Part model, mm, in its own coordinate system. A direction names the side the tool comes from. Coordinates: 2 decimals unless noted, no trailing zeros. Write each loop counter-clockwise with the first axis right and the second up, starting at its lowest first coordinate (ties: lowest second). Pieces come first, ordered by that corner, then holes. Notation, with made-up numbers: (89.5, -37.5) -> (113.5, -37.5) arc R17 cw to (113.5, -8.5) -> close; hole circle Ø3 at (70, 34.25). An arc over 180 degrees is marked (long way). One line per question, with ' | ' between items. Start each with the question number.
Item 1: Probe probe 1 along Y at (x, z) = (27, 27); probe 2 along Z at (x, y) = (30, 3.35); probe 3 along Y at (x, z) = (32, 24.5). List the from-to ranges inside material, lowest first. Write a range as [from, to].
Item 2: Two-plate mould, pull along Z, no slides. Class faces 4 (the cylindrical face through (18.894, 23.26, -27.671)), 5 (the flat face through (20, 0, -25)), 6 (the flat face through (20, 0, 25)): pulls with the +Z half, pulls with the -Z half, needs draft (parallel to the pull), parting line crosses it, or undercut.
Item 3: Saw through at C-C (y = 10). List the corners of the cut face in (x, z), and give its area (3 significant figures).
Item 4: Saw through at B-B (x = 30). Count the separate pieces of the cut face and the enclosed holes in it, and give its area (3 significant figures).
Item 5: Saw through at A-A (y = -13). List the corners of the cut face in (x, z), and give its area (3 significant figures).
Item 6: 3-axis set-ups, long thin cutter, end or side, ignore diameter. For faces 1 (the flat face through (20, -6, -11)), 2 (the flat face through (20, 33, 4.5)), 3 (the cylindrical face through (9.675, -36.464, -3.12)): which of +Z, -Z, +X, -X, +Y, -Y reach the whole face in a straight line?
Item 7: Pin check, flat tips, straight feed: pin 1 (3.5 mm diameter, centred on x = 10, y = 35, fed in from +Z); pin 2 (3 mm diameter, centred on x = 17, y = -35, fed in from -Z); pin 3 (4 mm diameter, centred on x = 8, z = 36, fed in from +Y). Stop position of each tip, or through.
from build123d import *

# Parameters (mm, degrees)
SKETCH1_R               = 17.5
SKETCH1_R_2             = 4.75
MAINBODY_DEPTH          = 40
SKETCH2_R               = 17.5
SKETCH2_R_2             = 11.25
BEARINGHOUSING_DEPTH    = 7.5
SKETCH3_R               = 1.5
MOUNTINGHOLES_DEPTH     = 20
BOSS_EXTRUDE3_DEPTH     = 40
SKETCH6_R               = 1.5
CUT_EXTRUDE2_DEPTH      = 10
FILLET1_R               = 5
CIRPATTERN1_DEPTH       = 40
CIRPATTERN1_START       = -5
CIRPATTERN1_2_OUTLINE_R = 1.5
CIRPATTERN1_2_DEPTH     = 10
CIRPATTERN1_3_OUTLINE_R = 1.5
CIRPATTERN1_3_DEPTH     = 10
CIRPATTERN1_4_OUTLINE_R = 1.5
CIRPATTERN1_4_DEPTH     = 10
CIRPATTERN1_5_OUTLINE_R = 1.5
CIRPATTERN1_5_DEPTH     = 10


with BuildPart() as part:
    # Sketch1 → MainBody (new body)
    with BuildSketch(Plane(origin=(0, 0, 0), x_dir=(0, 0, -1), z_dir=(1, 0, 0))):
        Circle(SKETCH1_R)
        Circle(SKETCH1_R_2, mode=Mode.SUBTRACT)
    extrude(amount=MAINBODY_DEPTH)

    # Sketch2 → BearingHousing (add)
    with BuildSketch(Plane(origin=(40, 0, 0), x_dir=(0, 0, -1), z_dir=(1, 0, 0))):
        Circle(SKETCH2_R)
        Circle(SKETCH2_R_2, mode=Mode.SUBTRACT)
    extrude(amount=BEARINGHOUSING_DEPTH)

    # Sketch3 → MountingHoles (cut)
    with BuildSketch(Plane.ZY):
        with Locations((0, 13)):
            Circle(SKETCH3_R)
        with Locations((11.258330249, 6.5)):
            Circle(SKETCH3_R)
        with Locations((11.258330249, -6.5)):
            Circle(SKETCH3_R)
        with Locations((0, -13)):
            Circle(SKETCH3_R)
        with Locations((-11.258330249, -6.5)):
            Circle(SKETCH3_R)
        with Locations((-11.258330249, 6.5)):
            Circle(SKETCH3_R)
    extrude(amount=-MOUNTINGHOLES_DEPTH, mode=Mode.SUBTRACT)

    # Sketch4 → Boss-Extrude3 (add)
    with BuildSketch(Plane.ZY):
        with BuildLine():
            Line((-4.5, 16.911534525), (-4.5, 45))
            Line((-4.5, 45), (-1.7, 45))
            Line((-1.7, 45), (-1.7, 25))
            Line((-1.7, 25), (1.7, 25))
            Line((1.7, 25), (1.7, 45))
            Line((1.7, 45), (4.5, 45))
            Line((4.5, 45), (4.5, 16.911534525))
            ThreePointArc((4.5, 16.911534525), (0, 17.5), (-4.5, 16.911534525))
        make_face()
    extrude(amount=-BOSS_EXTRUDE3_DEPTH)

    # Sketch6 → Cut-Extrude2 (cut)
    with BuildSketch(Plane(origin=(0, 0, -4.5), x_dir=(-1, 0, 0), z_dir=(0, 0, -1))):
        with Locations((-30, 35)):
            Circle(SKETCH6_R)
        with Locations((-20, 35)):
            Circle(SKETCH6_R)
        with Locations((-10, 35)):
            Circle(SKETCH6_R)
    extrude(amount=-CUT_EXTRUDE2_DEPTH, mode=Mode.SUBTRACT)

    # Fillet1
    fillet1_edges = [part.edges().sort_by_distance(p)[0] for p in [
        (20, 16.911534525, 4.5),
        (20, 16.911534525, -4.5),
    ]]
    fillet(fillet1_edges, radius=FILLET1_R)

    # CirPattern1: read off the stored shape, not the designer's step
    # CirPattern1 outline → CirPattern1 (add)
    with BuildSketch(Plane.YZ):
        with BuildLine():
            Line((-45, 4.5), (-45, 1.7))
            Line((-45, 1.7), (-25, 1.7))
            Line((-25, 1.7), (-25, -1.7))
            Line((-25, -1.7), (-45, -1.7))
            Line((-45, -1.7), (-45, -4.5))
            Line((-45, -4.5), (-20.396078054, -4.5))
            ThreePointArc((-20.396078054, -4.5), (-18.037369477, -5.091316086), (-16.236557831, -6.72540246))
            ThreePointArc((-16.236557831, -6.72540246), (-16.354450402, -9.154242143), (-17.604185617, -11.240224587))
            Line((-17.604185617, -11.240224587), (-35.001785669, -28.637824638))
            Line((-35.001785669, -28.637824638), (-33.021886681, -30.617723625))
            Line((-33.021886681, -30.617723625), (-18.879751058, -16.475588002))
            Line((-18.879751058, -16.475588002), (-16.475588002, -18.879751058))
            Line((-16.475588002, -18.879751058), (-30.617723625, -33.021886681))
            Line((-30.617723625, -33.021886681), (-28.637824638, -35.001785669))
            Line((-28.637824638, -35.001785669), (-11.240224587, -17.604185617))
            ThreePointArc((-11.240224587, -17.604185617), (-9.154242143, -16.354450402), (-6.72540246, -16.236557831))
            ThreePointArc((-6.72540246, -16.236557831), (-5.091316086, -18.037369477), (-4.5, -20.396078054))
            Line((-4.5, -20.396078054), (-4.5, -45))
            Line((-4.5, -45), (-1.7, -45))
            Line((-1.7, -45), (-1.7, -25))
            Line((-1.7, -25), (1.7, -25))
            Line((1.7, -25), (1.7, -45))
            Line((1.7, -45), (4.5, -45))
            Line((4.5, -45), (4.5, -20.396078054))
            ThreePointArc((4.5, -20.396078054), (5.091316086, -18.037369477), (6.72540246, -16.236557831))
            ThreePointArc((6.72540246, -16.236557831), (9.154242143, -16.354450402), (11.240224587, -17.604185617))
            Line((11.240224587, -17.604185617), (28.637824638, -35.001785669))
            Line((28.637824638, -35.001785669), (30.617723625, -33.021886681))
            Line((30.617723625, -33.021886681), (16.475588002, -18.879751058))
            Line((16.475588002, -18.879751058), (18.879751058, -16.475588002))
            Line((18.879751058, -16.475588002), (33.021886681, -30.617723625))
            Line((33.021886681, -30.617723625), (35.001785669, -28.637824638))
            Line((35.001785669, -28.637824638), (17.604185617, -11.240224587))
            ThreePointArc((17.604185617, -11.240224587), (16.354450402, -9.154242143), (16.236557831, -6.72540246))
            ThreePointArc((16.236557831, -6.72540246), (16.037443935, -7.05003906), (15.863616265, -7.388888889))
            ThreePointArc((15.863616265, -7.388888889), (-17.5, 0), (15.863616265, 7.388888889))
            ThreePointArc((15.863616265, 7.388888889), (16.037443935, 7.05003906), (16.236557831, 6.72540246))
            ThreePointArc((16.236557831, 6.72540246), (16.354450402, 9.154242143), (17.604185617, 11.240224587))
            Line((17.604185617, 11.240224587), (35.001785669, 28.637824638))
            Line((35.001785669, 28.637824638), (33.021886681, 30.617723625))
            Line((33.021886681, 30.617723625), (18.879751058, 16.475588002))
            Line((18.879751058, 16.475588002), (16.475588002, 18.879751058))
            Line((16.475588002, 18.879751058), (30.617723625, 33.021886681))
            Line((30.617723625, 33.021886681), (28.637824638, 35.001785669))
            Line((28.637824638, 35.001785669), (11.240224587, 17.604185617))
            ThreePointArc((11.240224587, 17.604185617), (9.154242143, 16.354450402), (6.72540246, 16.236557831))
            ThreePointArc((6.72540246, 16.236557831), (5.091316086, 18.037369477), (4.5, 20.396078054))
            Line((4.5, 20.396078054), (4.5, 45))
            Line((4.5, 45), (1.7, 45))
            Line((1.7, 45), (1.7, 25))
            Line((1.7, 25), (-1.7, 25))
            Line((-1.7, 25), (-1.7, 45))
            Line((-1.7, 45), (-4.5, 45))
            Line((-4.5, 45), (-4.5, 20.396078054))
            ThreePointArc((-4.5, 20.396078054), (-5.091316086, 18.037369477), (-6.72540246, 16.236557831))
            ThreePointArc((-6.72540246, 16.236557831), (-9.154242143, 16.354450402), (-11.240224587, 17.604185617))
            Line((-11.240224587, 17.604185617), (-28.637824638, 35.001785669))
            Line((-28.637824638, 35.001785669), (-30.617723625, 33.021886681))
            Line((-30.617723625, 33.021886681), (-16.475588002, 18.879751058))
            Line((-16.475588002, 18.879751058), (-18.879751058, 16.475588002))
            Line((-18.879751058, 16.475588002), (-33.021886681, 30.617723625))
            Line((-33.021886681, 30.617723625), (-35.001785669, 28.637824638))
            Line((-35.001785669, 28.637824638), (-17.604185617, 11.240224587))
            ThreePointArc((-17.604185617, 11.240224587), (-16.354450402, 9.154242143), (-16.236557831, 6.72540246))
            ThreePointArc((-16.236557831, 6.72540246), (-18.037369477, 5.091316086), (-20.396078054, 4.5))
            Line((-20.396078054, 4.5), (-45, 4.5))
        make_face()
    extrude(amount=CIRPATTERN1_DEPTH)

    # CirPattern1 2 outline → CirPattern1 2 (cut)
    with BuildSketch(Plane(origin=(0, 0, 0), x_dir=(1, 0, 0), z_dir=(0, 0.707106781186539, 0.707106781186556)).offset(CIRPATTERN1_START)):
        with Locations((30, 35)):
            Circle(CIRPATTERN1_2_OUTLINE_R)
        with Locations((20, 35)):
            Circle(CIRPATTERN1_2_OUTLINE_R)
        with Locations((10, 35)):
            Circle(CIRPATTERN1_2_OUTLINE_R)
        with Locations((10, -35)):
            Circle(CIRPATTERN1_2_OUTLINE_R)
        with Locations((20, -35)):
            Circle(CIRPATTERN1_2_OUTLINE_R)
        with Locations((30, -35)):
            Circle(CIRPATTERN1_2_OUTLINE_R)
    extrude(amount=CIRPATTERN1_2_DEPTH, mode=Mode.SUBTRACT)

    # CirPattern1 3 outline → CirPattern1 3 (cut)
    with BuildSketch(Plane(origin=(0, 0, 0), x_dir=(1, 0, 0), z_dir=(0, 1, 0)).offset(CIRPATTERN1_START)):
        with Locations((10, 35)):
            Circle(CIRPATTERN1_3_OUTLINE_R)
        with Locations((30, 35)):
            Circle(CIRPATTERN1_3_OUTLINE_R)
        with Locations((20, 35)):
            Circle(CIRPATTERN1_3_OUTLINE_R)
        with Locations((30, -35)):
            Circle(CIRPATTERN1_3_OUTLINE_R)
        with Locations((20, -35)):
            Circle(CIRPATTERN1_3_OUTLINE_R)
        with Locations((10, -35)):
            Circle(CIRPATTERN1_3_OUTLINE_R)
    extrude(amount=CIRPATTERN1_3_DEPTH, mode=Mode.SUBTRACT)

    # CirPattern1 4 outline → CirPattern1 4 (cut)
    with BuildSketch(Plane(origin=(0, 0, 0), x_dir=(1, 0, 0), z_dir=(0, 0.707106781186554, -0.707106781186541)).offset(CIRPATTERN1_START)):
        with Locations((30, 35)):
            Circle(CIRPATTERN1_4_OUTLINE_R)
        with Locations((20, 35)):
            Circle(CIRPATTERN1_4_OUTLINE_R)
        with Locations((10, 35)):
            Circle(CIRPATTERN1_4_OUTLINE_R)
        with Locations((30, -35)):
            Circle(CIRPATTERN1_4_OUTLINE_R)
        with Locations((20, -35)):
            Circle(CIRPATTERN1_4_OUTLINE_R)
        with Locations((10, -35)):
            Circle(CIRPATTERN1_4_OUTLINE_R)
    extrude(amount=CIRPATTERN1_4_DEPTH, mode=Mode.SUBTRACT)

    # CirPattern1 5 outline → CirPattern1 5 (cut)
    with BuildSketch(Plane.XY.offset(CIRPATTERN1_START)):
        with Locations((10, -35)):
            Circle(CIRPATTERN1_5_OUTLINE_R)
        with Locations((20, -35)):
            Circle(CIRPATTERN1_5_OUTLINE_R)
        with Locations((30, -35)):
            Circle(CIRPATTERN1_5_OUTLINE_R)
    extrude(amount=CIRPATTERN1_5_DEPTH, mode=Mode.SUBTRACT)


solid = part.part
From the geometry:
1) probe 1: [-33.36, -29.4], [-24.6, -20.64], [-4.5, -1.7], [1.7, 4.5], [20.64, 24.6], [29.4, 33.36] | probe 2: [-45, -36.5], [-33.5, -3.37], [3.37, 33.5], [36.5, 45] | probe 3: [-30.86, -26.9], [-22.1, -18.14], [-4.5, 4.5], [18.14, 22.1], [26.9, 30.86]
2) face 4: undercut | face 5: pulls with the -Z half | face 6: pulls with the +Z half
3) outline: (0, -16.7) -> (40, -16.7) -> (40, -14.36) -> (47.5, -14.36) -> (47.5, -5.15) -> (40, -5.15) -> (40, 5.15) -> (47.5, 5.15) -> (47.5, 14.36) -> (40, 14.36) -> (40, 16.7) -> (0, 16.7) -> close | area: 1,470 mm2
4) separate pieces: 17 | enclosed holes: 1 | area: 2,240 mm2
5) outline: (0, -19.36) -> (40, -19.36) -> (40, -11.72) -> (47.5, -11.72) -> (47.5, 11.72) -> (40, 11.72) -> (40, 19.36) -> (0, 19.36) -> (0, 1.5) -> (20, 1.5) -> (20, -1.5) -> (0, -1.5) -> close | area: 1,660 mm2
6) face 1: -X | face 2: +X, -X, +Y | face 3: none
7) pin 1: z = 30.39 | pin 2: z = -30.14 | pin 3: y = 29.64
